Part model, mm, in its own coordinate system. Coordinates: 2 decimals unless noted, no trailing zeros. Write each loop counter-clockwise with the first axis right and the second up, starting at its lowest first coordinate (ties: lowest second). Pieces come first, ordered by that corner, then holes. Notation, with made-up numbers: (78, 16.5) -> (113, 16.5) arc R11 ccw to (113, 26.5) -> close; hole circle Ø11 at (85, 64). An arc over 180 degrees is marked (long way). One line per question, with ' | ' between items. Start each with the question number.
Item 1: Saw through at B-B (x = 0.85). List the corners of the cut face in (y, z).
Item 2: Two-plate mould, pull along Y, no slides. Class faces 1 (the flat face through (0, 5, 76)), 2 (the cylindrical face through (1.48, 4.65, 146.56)), 3 (the flat face through (1, 10, 74)): pulls with the +Y half, pulls with the -Y half, needs draft (parallel to the pull), parting line crosses it, or undercut.
Item 3: Probe probe 1 along Z at (x, y) = (2.05, 5); probe 2 along Y at (x, z) = (1.1, 145); probe 3 along Z at (x, y) = (2.45, 2.75). List the from-to ranges inside material, lowest first. Write a range as [from, to].
Item 4: Saw through at A-A (y = 5). List the corners of the cut face in (x, z).
Autodesk Inventor part; units mm, degrees
ref_plane "YZ Plane" through (0, 0, 0) normal (1, 0, 0) x (0, 1, 0)
ref_plane "XZ Plane" through (0, 0, 0) normal (0, 1, 0) x (-1, 0, 0)
ref_plane "XY Plane" through (0, 0, 0) normal (0, 0, 1) x (1, 0, 0)
sketch "Szkic1" plane through (0, 0, 0) normal (1, 0, 0) x (0, 1, 0)
  line L0 (5, 0) -> (5, 0)
  line L1 (10, 5) -> (10, 145)
  line L2 (5, 150) -> (5, 150)
  line L3 (0, 145) -> (0, 5)
  arc A0 (10, 145) -> (5, 150) centre (5, 145) ccw
  arc A1 (5, 150) -> (0, 145) centre (5, 145) ccw
  arc A2 (5, 0) -> (10, 5) centre (5, 5) ccw
  arc A3 (0, 5) -> (5, 0) centre (5, 5) ccw
  circle A4 centre (5, 145) radius 1.6
  circle A5 centre (5, 5) radius 1.6
  point P0 (0, 0)
  point P1 (10, 150)
  point P2 (0, 150)
  dimension "d0" = 10
  dimension "d1" = 5
  dimension "d2" = 140
  dimension "d3" = 3.2
  dimension "d4" = 3.2
extrude "Wyciągnięcie proste1" add sketch "Szkic1" along normal blind 3
properties part number "korbowód"
From the geometry:
1) outline: (0, 5) arc R5 ccw to (10, 5) -> (10, 145) arc R5 ccw to (0, 145) -> close; hole circle Ø3.2 at (5, 5); hole circle Ø3.2 at (5, 145)
2) face 1: needs draft | face 2: undercut | face 3: pulls with the +Y half
3) probe 1: [0, 3.4], [6.6, 143.4], [146.6, 150] | probe 2: [0, 3.4], [6.6, 10] | probe 3: [0.53, 149.47]
4) outline: (0, 0) -> (3, 0) -> (3, 3.4) -> (0, 3.4) -> close; (0, 6.6) -> (3, 6.6) -> (3, 143.4) -> (0, 143.4) -> close; (0, 146.6) -> (3, 146.6) -> (3, 150) -> (0, 150) -> close
